Geometry check sheet. Reference: the model listing, model coordinates, mm. A direction names the side the tool comes from. Give positions to 0.01 mm unless a question says otherwise; leave off trailing zeros. Write each loop counter-clockwise with the first axis right and the second up, starting at its lowest first coordinate (ties: lowest second). Pieces come first, ordered by that corner, then holes. Notation, with made-up numbers: (42.25, -1) - (59.25, -1) arc R27 cw to (59.25, 18) - close; hole circle Ø3 at (-12, -19.5). An arc over 180 degrees is marked (long way). Write item = value, one per line. Start each with the question number.
(1) Thickness scan on L1, parallel to Z at x = 36, y = 42.5; L2, parallel to X at y = 184.5, z = 72; L3, parallel to Y at x = 7, z = 48. Record the ranges inside material, lowest first.
(2) Section check A-A, the plane y = 275. Enter the section's corners in (x, z).
(3) Access from +Z, -Z, +X, -X, +Y, -Y to the whole of each face (thin tool, end or side, straight path). Record for faces 1 (the flat face through (18, 184, -117.208)), 2 (the cylindrical face through (-62.563, 183.495, -131.412)), 3 (the cylindrical face through (100.02, 183.5, 206.17)).
(4) Draft check along Y on faces 4 (the flat face through (18, 179, -134.988)), 5 (the flat face through (-58, 354.584, 24)), 6 (the flat face through (92.162, 184, 40)). Enter one of: pulls with the +Y half, pulls with the -Y half, needs draft (parallel to the pull), parting line crosses it, or undercut.
(5) Section check B-B, the plane z = 150.5. Enter the section's corners in (x, y), plus the area to 3 significant figures.
(6) Section check C-C, the plane x = 19.5. Enter the section's corners in (y, z).
(7) Depth check by flat-ended pin: pin 1 Ø3 at (x, y) = (-1, 353.5) entering from -Z; pin 2 Ø5 at (x, y) = (66.5, 38.5) entering from -Z; pin 3 Ø4 at (x, y) = (68, 193) entering from +Z. Enter the tip coordinate at first touch or a pass-through.
```python
from build123d import *

# Parameters (mm, degrees)
SKETCH1_W            = 169.926
SKETCH1_H            = 344.932
BOSS_EXTRUDE1_DEPTH  = 379.984
SKETCH7_W            = 344.932
SKETCH7_H            = 10.16
BOSS_EXTRUDE4_DEPTH  = 2.54
SKETCH8_W            = 344.932
SKETCH8_H            = 10.16
BOSS_EXTRUDE5_DEPTH  = 2.54
SKETCH9_W            = 175.006
SKETCH9_H            = 10.16
BOSS_EXTRUDE6_DEPTH  = 2.54
SKETCH13_W           = 344.932
SKETCH13_H           = 2.54
BOSS_EXTRUDE9_DEPTH  = 1.27
SKETCH14_W           = 171.196
SKETCH14_H           = 2.54
BOSS_EXTRUDE10_DEPTH = 1.27
SKETCH15_W           = 346.202
SKETCH15_H           = 2.54
BOSS_EXTRUDE11_DEPTH = 1.27
SKETCH16_W           = 172.466
SKETCH16_H           = 2.54
BOSS_EXTRUDE12_DEPTH = 1.27
FILLET1_R            = 12.54
SKETCH23_W           = 175.014872456
SKETCH23_H           = 10.16
BOSS_EXTRUDE15_DEPTH = 2.54
SKETCH25_W           = 180.28813578
SKETCH25_H           = 28.656047844
CUT_EXTRUDE1_DEPTH   = 474.472
SKETCH26_W           = 147.066
SKETCH26_H           = 309.372
CUT_EXTRUDE2_DEPTH   = 345.948


with BuildPart() as part:
    # Sketch1 → Boss-Extrude1 (new body)
    with BuildSketch(Plane(origin=(0, 0, 0), x_dir=(1, 0, 0), z_dir=(0, 1, 0))):
        with Locations((18.629158276, -37.477981942)):
            Rectangle(SKETCH1_W, SKETCH1_H)
    extrude(amount=BOSS_EXTRUDE1_DEPTH)

    # Sketch7 → Boss-Extrude4 (add)
    with BuildSketch(Plane.ZY.offset(66.333841724)):
        with Locations((37.477981942, 5.08)):
            Rectangle(SKETCH7_W, SKETCH7_H)
    extrude(amount=BOSS_EXTRUDE4_DEPTH)

    # Sketch8 → Boss-Extrude5 (add)
    with BuildSketch(Plane(origin=(103.592158276, 0, 0), x_dir=(0, 0, -1), z_dir=(1, 0, 0))):
        with Locations((-37.477981942, 5.08)):
            Rectangle(SKETCH8_W, SKETCH8_H)
    extrude(amount=BOSS_EXTRUDE5_DEPTH)

    # Sketch9 → Boss-Extrude6 (add)
    with BuildSketch(Plane(origin=(0, 0, -134.988018058), x_dir=(-1, 0, 0), z_dir=(0, 0, -1))):
        with Locations((-18.629158276, 5.08)):
            Rectangle(SKETCH9_W, SKETCH9_H)
    extrude(amount=BOSS_EXTRUDE6_DEPTH)

    # Sketch13 → Boss-Extrude9 (add)
    with BuildSketch(Plane(origin=(103.592158276, 0, 0), x_dir=(0, 0, -1), z_dir=(1, 0, 0))):
        with Locations((-37.477981942, 353.314)):
            Rectangle(SKETCH13_W, SKETCH13_H)
    extrude(amount=BOSS_EXTRUDE9_DEPTH)

    # Sketch14 → Boss-Extrude10 (add)
    with BuildSketch(Plane(origin=(0, 0, -134.988018058), x_dir=(-1, 0, 0), z_dir=(0, 0, -1))):
        with Locations((-19.264158276, 353.314)):
            Rectangle(SKETCH14_W, SKETCH14_H)
    extrude(amount=BOSS_EXTRUDE10_DEPTH)

    # Sketch15 → Boss-Extrude11 (add)
    with BuildSketch(Plane.ZY.offset(66.333841724)):
        with Locations((36.842981942, 353.314)):
            Rectangle(SKETCH15_W, SKETCH15_H)
    extrude(amount=BOSS_EXTRUDE11_DEPTH)

    # Sketch16 → Boss-Extrude12 (add)
    with BuildSketch(Plane.XY.offset(209.943981942)):
        with Locations((18.629158276, 353.314)):
            Rectangle(SKETCH16_W, SKETCH16_H)
    extrude(amount=BOSS_EXTRUDE12_DEPTH)

    # Fillet1
    fillet1_edges = [part.edges().sort_by_distance(p)[0] for p in [
        (103.592158276, 379.984, 37.477981942),
        (18.629158276, 379.984, -134.988018058),
        (-66.333841724, 379.984, 37.477981942),
        (103.592158276, 181.102, 209.943981942),
        (103.592158276, 181.102, -134.988018058),
        (-66.333841724, 181.102, -134.988018058),
        (-66.333841724, 367.284, -134.988018058),
        (103.592158276, 367.284, -134.988018058),
        (103.592158276, 367.284, 209.943981942),
        (-66.333841724, 367.284, 209.943981942),
        (-66.333841724, 181.102, 209.943981942),
        (18.629158276, 379.984, 209.943981942),
    ]]
    fillet(fillet1_edges, radius=FILLET1_R)

    # Sketch23 → Boss-Extrude15 (add)
    with BuildSketch(Plane.XY.offset(209.943981942)):
        with Locations((18.633594504, 5.08)):
            Rectangle(SKETCH23_W, SKETCH23_H)
    extrude(amount=BOSS_EXTRUDE15_DEPTH)

    # Sketch25 → Cut-Extrude1 (cut)
    with BuildSketch(Plane(origin=(0, 0, -134.988018058), x_dir=(-1, 0, 0), z_dir=(0, 0, -1))):
        with Locations((-13.448090386, 368.912023922)):
            Rectangle(SKETCH25_W, SKETCH25_H)
    extrude(amount=-CUT_EXTRUDE1_DEPTH, mode=Mode.SUBTRACT)

    # Sketch26 → Cut-Extrude2 (cut)
    with BuildSketch(Plane(origin=(0, 354.584, 0), x_dir=(1, 0, 0), z_dir=(0, 1, 0))):
        with Locations((18.629158276, -37.477981942)):
            Rectangle(SKETCH26_W, SKETCH26_H)
    extrude(amount=-CUT_EXTRUDE2_DEPTH, mode=Mode.SUBTRACT)


solid = part.part
```
Model answer:
q1.L1 = -134.99 to -117.21, 192.16 to 209.94
q1.L2 = -66.33 to -54.9, 92.16 to 103.59
q1.L3 = 0 to 8.64
q2.outline = (-66.33, -122.45) arc R12.54 ccw to (-53.79, -134.99) - (91.05, -134.99) arc R12.54 ccw to (103.59, -122.45) - (103.59, 197.4) arc R12.54 ccw to (91.05, 209.94) - (-53.79, 209.94) arc R12.54 ccw to (-66.33, 197.4) - close; hole (-54.9, -117.21) - (92.16, -117.21) - (92.16, 192.16) - (-54.9, 192.16) - close
q3.face_1 = +Y
q3.face_2 = -Z, -X
q3.face_3 = +Z, +X
q4.face_4 = undercut
q4.face_5 = pulls with the +Y half
q4.face_6 = needs draft
q5.outline = (-68.87, 0) - (106.13, 0) - (106.13, 10.16) - (103.59, 10.16) - (103.59, 352.04) - (104.86, 352.04) - (104.86, 354.58) - (92.16, 354.58) - (92.16, 8.64) - (-54.9, 8.64) - (-54.9, 354.58) - (-67.6, 354.58) - (-67.6, 352.04) - (-66.33, 352.04) - (-66.33, 10.16) - (-68.87, 10.16) - close
q5.area = 9,430 mm²
q6.outline = (0, -137.53) - (10.16, -137.53) - (10.16, -134.99) - (352.04, -134.99) - (352.04, -136.26) - (354.58, -136.26) - (354.58, -117.21) - (8.64, -117.21) - (8.64, 192.16) - (354.58, 192.16) - (354.58, 211.21) - (352.04, 211.21) - (352.04, 209.94) - (10.16, 209.94) - (10.16, 212.48) - (0, 212.48) - close
q7.pin_1 = -136.26
q7.pin_2 = -134.99
q7.pin_3 = 209.94
